```python
from build123d import *

# Parameters (mm, degrees)
SKETCH1_W            = 8.5
SKETCH1_H            = 22
BOSS_EXTRUDE1_DEPTH  = 5
CUT_EXTRUDE1_DEPTH   = 3.5
SKETCH3_R            = 1.5
CUT_EXTRUDE2_DEPTH   = 1.5
SKETCH4_W            = 8.5
SKETCH4_H            = 6
BOSS_EXTRUDE2_DEPTH  = 23
SKETCH7_W            = 8.5
SKETCH7_H            = 22
BOSS_EXTRUDE4_DEPTH  = 5
CUT_EXTRUDE3_DEPTH   = 3.5
SKETCH9_R            = 1.5
CUT_EXTRUDE4_DEPTH   = 3.5
SKETCH10_W           = 8.5
SKETCH10_H           = 6
BOSS_EXTRUDE5_DEPTH  = 23
SKETCH6_W            = 6
SKETCH6_H            = 8
BOSS_EXTRUDE6_DEPTH  = 30.5
SKETCH11_W           = 47.5
SKETCH11_H           = 8
BOSS_EXTRUDE7_DEPTH  = 13.5
SKETCH12_W           = 47.5
SKETCH12_H           = 8
BOSS_EXTRUDE8_DEPTH  = 5.5
SKETCH13_W           = 5
SKETCH13_H           = 6
CUT_EXTRUDE5_DEPTH   = 15
SKETCH14_W           = 5
SKETCH14_H           = 6
CUT_EXTRUDE6_DEPTH   = 4
SKETCH15_W           = 5
SKETCH15_H           = 6
CUT_EXTRUDE7_DEPTH   = 15
SKETCH16_W           = 5
SKETCH16_H           = 6
CUT_EXTRUDE8_DEPTH   = 4
SKETCH17_W           = 5
SKETCH17_H           = 6
BOSS_EXTRUDE9_DEPTH  = 2
SKETCH18_W           = 10.5
SKETCH18_H           = 8
BOSS_EXTRUDE10_DEPTH = 5
CUT_EXTRUDE9_DEPTH   = 2
SKETCH23_R           = 1.5
CUT_EXTRUDE10_DEPTH  = 3.5
CUT_EXTRUDE11_REACH  = 58.867
SKETCH24_R           = 1.5
SKETCH25_W           = 5
SKETCH25_H           = 6
BOSS_EXTRUDE11_DEPTH = 2


with BuildPart() as part:
    # Sketch1 → Boss-Extrude1 (new body)
    with BuildSketch(Plane(origin=(0, 0, 0), x_dir=(1, 0, 0), z_dir=(0, 1, 0))):
        Rectangle(SKETCH1_W, SKETCH1_H)
    extrude(amount=BOSS_EXTRUDE1_DEPTH)

    # Sketch2 → Cut-Extrude1 (cut)
    with BuildSketch(Plane(origin=(0, 5, 0), x_dir=(1, 0, 0), z_dir=(0, 1, 0))):
        Polygon((-1.705, 9.703146627), (-3.41, 6.75), (-1.705, 3.796853373), (1.705, 3.796853373), (3.41, 6.75), (1.705, 9.703146627), align=None)
        Polygon((1.705, -9.703146627), (-1.705, -9.703146627), (-3.41, -6.75), (-1.705, -3.796853373), (1.705, -3.796853373), (3.41, -6.75), align=None)
    extrude(amount=-CUT_EXTRUDE1_DEPTH, mode=Mode.SUBTRACT)

    # Sketch3 → Cut-Extrude2 (cut)
    with BuildSketch(Plane(origin=(0, 1.5, 0), x_dir=(1, 0, 0), z_dir=(0, 1, 0))):
        with Locations(Location((0, 6.75, 0), (0, 0, 270))):
            Circle(SKETCH3_R)
        with Locations(Location((0, -6.75, 0), (0, 0, 270))):
            Circle(SKETCH3_R)
        with Locations((39, 6.75)):
            Circle(SKETCH3_R)
        with Locations((39, -6.75)):
            Circle(SKETCH3_R)
    extrude(amount=-CUT_EXTRUDE2_DEPTH, mode=Mode.SUBTRACT)

    # Sketch4 → Boss-Extrude2 (add)
    with BuildSketch(Plane(origin=(0, 5, 0), x_dir=(1, 0, 0), z_dir=(0, 1, 0))):
        Rectangle(SKETCH4_W, SKETCH4_H)
    extrude(amount=BOSS_EXTRUDE2_DEPTH)



with BuildPart() as body_2:
    # Sketch7 → Boss-Extrude4 (new body)
    with BuildSketch(Plane(origin=(0, 0, 0), x_dir=(1, 0, 0), z_dir=(0, 1, 0))):
        with Locations((39, 0)):
            Rectangle(SKETCH7_W, SKETCH7_H)
    extrude(amount=BOSS_EXTRUDE4_DEPTH)

    # Sketch8 → Cut-Extrude3 (cut)
    with BuildSketch(Plane(origin=(0, 5, 0), x_dir=(1, 0, 0), z_dir=(0, 1, 0))):
        Polygon((40.705, 9.703146627), (37.295, 9.703146627), (35.59, 6.75), (37.295, 3.796853373), (40.705, 3.796853373), (42.41, 6.75), align=None)
        Polygon((40.705, -3.796853373), (37.295, -3.796853373), (35.59, -6.75), (37.295, -9.703146627), (40.705, -9.703146627), (42.41, -6.75), align=None)
    extrude(amount=-CUT_EXTRUDE3_DEPTH, mode=Mode.SUBTRACT)

    # Sketch9 → Cut-Extrude4 (cut)
    with BuildSketch(Plane(origin=(0, 1.5, 0), x_dir=(1, 0, 0), z_dir=(0, 1, 0))):
        with Locations(Location((39, 6.75, 0), (0, 0, 270))):
            Circle(SKETCH9_R)
        with Locations(Location((39, -6.75, 0), (0, 0, 270))):
            Circle(SKETCH9_R)
    extrude(amount=-CUT_EXTRUDE4_DEPTH, mode=Mode.SUBTRACT)

    # Sketch10 → Boss-Extrude5 (add)
    with BuildSketch(Plane(origin=(0, 5, 0), x_dir=(1, 0, 0), z_dir=(0, 1, 0))):
        with Locations((39, 0)):
            Rectangle(SKETCH10_W, SKETCH10_H)
    extrude(amount=BOSS_EXTRUDE5_DEPTH)


with BuildPart() as part_1:
    add(part.part)

    add(body_2.part)  # Boss-Extrude6 merges body 2
    # Sketch6 → Boss-Extrude6 (add)
    with BuildSketch(Plane(origin=(4.25, 0, 0), x_dir=(0, 0, -1), z_dir=(1, 0, 0))):
        with Locations((0, 24)):
            Rectangle(SKETCH6_W, SKETCH6_H)
    extrude(amount=BOSS_EXTRUDE6_DEPTH)

    # Sketch11 → Boss-Extrude7 (add)
    with BuildSketch(Plane(origin=(0, 0, -3), x_dir=(-1, 0, 0), z_dir=(0, 0, -1))):
        with Locations((-19.5, 24)):
            Rectangle(SKETCH11_W, SKETCH11_H)
    extrude(amount=BOSS_EXTRUDE7_DEPTH)

    # Sketch12 → Boss-Extrude8 (add)
    with BuildSketch(Plane(origin=(0, 0, -16.5), x_dir=(-1, 0, 0), z_dir=(0, 0, -1))):
        with Locations((-19.5, 24)):
            Rectangle(SKETCH12_W, SKETCH12_H)
    extrude(amount=BOSS_EXTRUDE8_DEPTH)

    # Sketch13 → Cut-Extrude5 (cut)
    with BuildSketch(Plane.ZY.offset(4.25)):
        with Locations((-16.5, 24)):
            Rectangle(SKETCH13_W, SKETCH13_H)
    extrude(amount=-CUT_EXTRUDE5_DEPTH, mode=Mode.SUBTRACT)

    # Sketch14 → Cut-Extrude6 (cut)
    with BuildSketch(Plane(origin=(0, 0, -22), x_dir=(-1, 0, 0), z_dir=(0, 0, -1))):
        with Locations((-8.25, 24)):
            Rectangle(SKETCH14_W, SKETCH14_H)
    extrude(amount=-CUT_EXTRUDE6_DEPTH, mode=Mode.SUBTRACT)

    # Sketch15 → Cut-Extrude7 (cut)
    with BuildSketch(Plane(origin=(43.25, 0, 0), x_dir=(0, 0, -1), z_dir=(1, 0, 0))):
        with Locations((16.5, 24)):
            Rectangle(SKETCH15_W, SKETCH15_H)
    extrude(amount=-CUT_EXTRUDE7_DEPTH, mode=Mode.SUBTRACT)

    # Sketch16 → Cut-Extrude8 (cut)
    with BuildSketch(Plane(origin=(0, 0, -22), x_dir=(-1, 0, 0), z_dir=(0, 0, -1))):
        with Locations((-32.75, 24)):
            Rectangle(SKETCH16_W, SKETCH16_H)
    extrude(amount=-CUT_EXTRUDE8_DEPTH, mode=Mode.SUBTRACT)

    # Sketch17 → Boss-Extrude9 (add)
    with BuildSketch(Plane(origin=(43.25, 0, 0), x_dir=(0, 0, -1), z_dir=(1, 0, 0))):
        Polygon((-3, 5), (-11, 5), (-11, 0), (11, 0), (11, 5), (3, 5), (3, 20), (22, 20), (22, 28), (-3, 28), align=None)
        with Locations((16.5, 24)):
            Rectangle(SKETCH17_W, SKETCH17_H, mode=Mode.SUBTRACT)
    extrude(amount=BOSS_EXTRUDE9_DEPTH)

    # Sketch18 → Boss-Extrude10 (add)
    with BuildSketch(Plane(origin=(0, 5, 0), x_dir=(1, 0, 0), z_dir=(0, 1, 0))):
        with Locations((40, -7)):
            Rectangle(SKETCH18_W, SKETCH18_H)
        with Locations((40, 7)):
            Rectangle(SKETCH18_W, SKETCH18_H)
    extrude(amount=-BOSS_EXTRUDE10_DEPTH)

    # Sketch20 → Cut-Extrude9 (cut)
    with BuildSketch(Plane.ZY.offset(-34.75)):
        Polygon((-3, 5), (-11, 5), (-11, 0), (11, 0), (11, 5), (3, 5), (3, 20), (-3, 20), align=None)
    extrude(amount=-CUT_EXTRUDE9_DEPTH, mode=Mode.SUBTRACT)

    # Sketch23 → Cut-Extrude10 (cut)
    with BuildSketch(Plane(origin=(0, 5, 0), x_dir=(1, 0, 0), z_dir=(0, 1, 0))):
        Polygon((42.705, 9.703146627), (39.295, 9.703146627), (37.59, 6.75), (39.295, 3.796853373), (42.705, 3.796853373), (44.41, 6.75), align=None)
        with Locations((41, 6.75)):
            Circle(SKETCH23_R, mode=Mode.SUBTRACT)
        with Locations((41, 6.75)):
            Circle(SKETCH23_R)
        Polygon((39.295, -9.703146627), (42.705, -9.703146627), (44.41, -6.75), (42.705, -3.796853373), (39.295, -3.796853373), (37.59, -6.75), align=None)
        with Locations((41, -6.75)):
            Circle(SKETCH23_R, mode=Mode.SUBTRACT)
        with Locations((41, -6.75)):
            Circle(SKETCH23_R)
    extrude(amount=-CUT_EXTRUDE10_DEPTH, mode=Mode.SUBTRACT)

    # Sketch24 → Cut-Extrude11 (cut, up to next)
    with BuildSketch(Plane(origin=(0, 1.5, 0), x_dir=(1, 0, 0), z_dir=(0, 1, 0)), mode=Mode.PRIVATE) as cut_extrude11_sk1:
        with Locations(Location((41, -6.75, 0), (0, 0, 270))):
            Circle(SKETCH24_R)
    cut_extrude11_tool1 = extrude(cut_extrude11_sk1.sketch, amount=-CUT_EXTRUDE11_REACH, mode=Mode.PRIVATE) & part_1.part
    # Sketch24 → Cut-Extrude11 (cut, up to next)
    with BuildSketch(Plane(origin=(0, 1.5, 0), x_dir=(1, 0, 0), z_dir=(0, 1, 0)), mode=Mode.PRIVATE) as cut_extrude11_sk2:
        with Locations(Location((41, 6.75, 0), (0, 0, 270))):
            Circle(SKETCH24_R)
    cut_extrude11_tool2 = extrude(cut_extrude11_sk2.sketch, amount=-CUT_EXTRUDE11_REACH, mode=Mode.PRIVATE) & part_1.part
    add(cut_extrude11_tool1.solids().sort_by_distance((41, 1.5, 6.75))[0], mode=Mode.SUBTRACT)
    add(cut_extrude11_tool2.solids().sort_by_distance((41, 1.5, -6.75))[0], mode=Mode.SUBTRACT)

    # Sketch25 → Boss-Extrude11 (add)
    with BuildSketch(Plane(origin=(28.25, 0, 0), x_dir=(0, 0, -1), z_dir=(1, 0, 0))):
        with Locations((16.5, 24)):
            Rectangle(SKETCH25_W, SKETCH25_H)
    extrude(amount=BOSS_EXTRUDE11_DEPTH)


solid = part_1.part
```
Read the model definition and answer for the solid it produces. Units are mm, in the model's axes. A direction names the side the tool comes from. Coordinates: 2 decimals unless noted, no trailing zeros. Loops run counter-clockwise (first coordinate to the right, second up) from the corner with the lowest first, then second, coordinate; pieces in that order, holes last. Notation, with made-up numbers: (67, 83.25) -> (78, 83.25) arc R24 ccw to (78, 111.25) -> close; hole circle Ø2 at (86.25, -3.5). An arc over 180 degrees is marked (long way). Return JSON: item names as keys, results as strings.
Item 1: For faces 1 (the flat face through (2.569, 3.274, 8.206)), 2 (the flat face through (2.546, 3.274, -5.253)), 3 (the flat face through (41, 5, -10)), determine the directions among +Z, -Z, +X, -X, +Y, -Y from which every point of the face is accessible in a straight line to the end or side of a thin tool.
Answers:
{"face 1": "+Y", "face 2": "none", "face 3": "-Z, +X, -X"}
Item 2: For a pull along X with two mould halves and no side action, classify faces 4 (the flat face through (41, 3, 11)), 5 (the flat face through (-2.569, 3.274, 5.294)) as +X half, -X half, draft (parallel to the pull), parting line (faces both ways), or undercut.
Answers:
{"face 4": "draft", "face 5": "undercut"}
Item 3: Flat-ended cylindrical pins translate along their axes: P1, Ø2.5, axis at x = 0, z = 6.75, coming from the +Y side; P2, Ø4.5, axis at x = 0.5, z = 7, coming from the +Y side; P3, Ø1.8, axis at x = -0.5, y = 23, coming from the +Z side; P4, Ø4, axis at x = 37, z = 1, coming from the -Y side. Find the tip coordinate at first contact, or state that the pin passes through.
Answers:
{"P1": "passes through", "P2": "stops at y = 1.5", "P3": "stops at z = 3", "P4": "stops at y = 0"}
Item 4: Find section D-D (x = 32). Determine the outline of the cut face in (y, z), plus the area to 3 significant figures.
Answers:
{"outline": "(20, -22) -> (21, -22) -> (21, -14) -> (27, -14) -> (27, -22) -> (28, -22) -> (28, 3) -> (20, 3) -> close", "area": "152 mm2"}
Item 5: Find section A-A (x = 41). Count the separate pieces of the cut face and the enclosed holes in it, plus the area to 3 significant figures.
Answers:
{"separate pieces": "3", "enclosed holes": "1", "area": "320 mm2"}
Item 6: Find the intervals of material crossed by probe 1 along X at (y, z) = (0.6, 6.75); probe 2 along Y at (x, z) = (41.5, -4.5); probe 3 along Z at (x, y) = (3, 25.25), in increasing order.
Answers:
{"probe 1": "x = -4.25 to -1.5, 1.5 to 4.25, 36.75 to 39.5, 42.5 to 45.25", "probe 2": "y = 0 to 1.5, 20 to 28", "probe 3": "z = -22 to -19, -14 to 3"}
Item 7: Find section C-C (z = -1). Determine the outline of the cut face in (x, y), plus the area to 3 significant figures.
Answers:
{"outline": "(-4.25, 0) -> (4.25, 0) -> (4.25, 20) -> (36.75, 20) -> (36.75, 0) -> (45.25, 0) -> (45.25, 28) -> (-4.25, 28) -> close", "area": "736 mm2"}
Item 8: Find section B-B (y = 14). Determine the outline of the cut face in (x, z).
Answers:
{"outline": "(-4.25, -3) -> (4.25, -3) -> (4.25, 3) -> (-4.25, 3) -> close; (36.75, -3) -> (45.25, -3) -> (45.25, 3) -> (36.75, 3) -> close"}
